The listing builds one solid part. Answer for the finished solid, in the listing's coordinates (mm). Face numbers are marked on the shaded views. A direction names the side the tool comes from. Give positions to 0.01 mm unless a question says otherwise; leave off trailing zeros. Order: outer loops, then holes, each group sorted by start corner. A loop starts at its lowest first (then second) coordinate and runs counter-clockwise, first axis right, second up. Notation, with made-up numbers: (46.5, -9) - (104.5, -9) arc R16 cw to (104.5, 0) - close; hole circle Ø10 at (40.25, 4). An arc over 180 degrees is marked (long way). Write each question's results on one line, items separated by ' | '. Start each with the question number.
1. Section D-D (x = 5) is taken. Give the vertices of the cut face in (y, z), and give its area (3 significant figures).
2. Determine the mould class of the marked faces 5, 6 and 7 for opening direction X: released by +X, released by -X, zero draft, split by the parting line, or undercut.
3. Find the intervals of material crossed by L1, parallel to Y at x = 0, z = 5.9; L2, parallel to X at y = 0, z = -9; L3, parallel to Z at x = -5.5, y = 4.5, in increasing order.
4. Section A-A (y = 0) is taken. Give the vertices of the cut face in (x, z), and give its area (3 significant figures).
5. Section C-C (z = -8) is taken. Give the vertices of the cut face in (x, y).
6. Section B-B (x = 0) is taken. Give the vertices of the cut face in (y, z).
7. Flat-ended cylindrical pins translate along their axes: pin 1 (4 mm diameter, centred on x = -4, z = -12.5, fed in from -Y); pin 2 (10 mm diameter, centred on x = -1.5, z = -9, fed in from +Y); pin 3 (4.5 mm diameter, centred on x = 0, y = 0, fed in from +Z). Find the tip coordinate at first contact, or state that the pin passes through.
8. Which of the six approach directions +Z, -Z, +X, -X, +Y, -Y give full straight-line access (tool end or side, diameter ignored) to the marked faces 1, 2, 3 and 4?
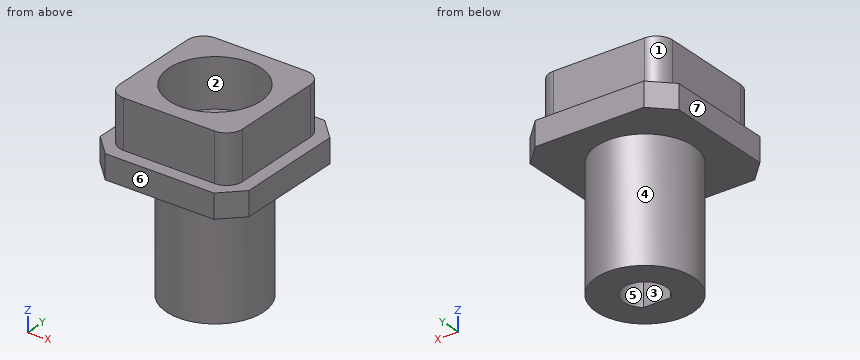
from build123d import *

# Parameters (mm, degrees)
PAD_DEPTH    = 3
SKETCH001_W  = 15.3
SKETCH001_H  = 15.3
SKETCH001_R  = 5.7
PAD001_DEPTH = 6
SKETCH002_R  = 6
PAD002_DEPTH = 15
POCKET_DEPTH = 24.001
FILLET_R     = 2


with BuildPart() as part:
    # Sketch → Pad (new body)
    with BuildSketch(Plane.XY):
        Polygon((-9.25, 6.75), (-6.75, 9.25), (6.75, 9.25), (9.25, 6.75), (9.25, -6.75), (6.75, -9.25), (-6.75, -9.25), (-9.25, -6.75), align=None)
    extrude(amount=PAD_DEPTH)

    # Sketch001 → Pad001 (new body)
    with BuildSketch(Plane.XY.offset(3)):
        Rectangle(SKETCH001_W, SKETCH001_H)
        Circle(SKETCH001_R, mode=Mode.SUBTRACT)
    extrude(amount=PAD001_DEPTH)

    # Sketch002 → Pad002 (new body)
    with BuildSketch(Plane(origin=(0, 0, 0), x_dir=(1, 0, 0), z_dir=(0, 0, -1))):
        Circle(SKETCH002_R)
    extrude(amount=PAD002_DEPTH)

    # Sketch003 → Pocket (cut, through all)
    with BuildSketch(Plane(origin=(0, 0, -15), x_dir=(1, 0, 0), z_dir=(0, 0, -1))):
        with BuildLine():
            Line((-1.684191, 2.02), (1.684191, 2.02))
            ThreePointArc((-1.684191, 2.02), (0, -2.63), (1.684191, 2.02))
        make_face()
    extrude(amount=-POCKET_DEPTH, mode=Mode.SUBTRACT)

    # Fillet
    fillet_edges = [part.edges().sort_by_distance(p)[0] for p in [
        (-7.65, -7.65, 6),
        (7.65, -7.65, 6),
        (-7.65, 7.65, 6),
        (7.65, 7.65, 6),
    ]]
    fillet(fillet_edges, radius=FILLET_R)


solid = part.part
Reported:
1) outline: (-9.25, 0) - (-3.32, 0) - (-3.32, -15) - (3.32, -15) - (3.32, 0) - (9.25, 0) - (9.25, 3) - (7.65, 3) - (7.65, 9) - (2.74, 9) - (2.74, 3) - (-2.74, 3) - (-2.74, 9) - (-7.65, 9) - (-7.65, 3) - (-9.25, 3) - close | area: 214 mm²
2) face 5: undercut | face 6: zero draft | face 7: released by -X
3) L1: -7.65 to -5.7, 5.7 to 7.65 | L2: -6 to -2.63, 2.63 to 6 | L3: 0 to 9
4) outline: (-9.25, 0) - (-6, 0) - (-6, -15) - (-2.63, -15) - (-2.63, 3) - (-5.7, 3) - (-5.7, 9) - (-7.65, 9) - (-7.65, 3) - (-9.25, 3) - close; (2.63, -15) - (6, -15) - (6, 0) - (9.25, 0) - (9.25, 3) - (7.65, 3) - (7.65, 9) - (5.7, 9) - (5.7, 3) - (2.63, 3) - close | area: 164 mm²
5) outline: circle Ø12 at (0, 0); hole (-1.68, -2.02) - (1.68, -2.02) arc R2.63 ccw (long way) to start
6) outline: (-9.25, 0) - (-6, 0) - (-6, -15) - (-2.02, -15) - (-2.02, 3) - (-5.7, 3) - (-5.7, 9) - (-7.65, 9) - (-7.65, 3) - (-9.25, 3) - close; (2.63, -15) - (6, -15) - (6, 0) - (9.25, 0) - (9.25, 3) - (7.65, 3) - (7.65, 9) - (5.7, 9) - (5.7, 3) - (2.63, 3) - close
7) pin 1: y = -5.66 | pin 2: y = 6 | pin 3: z = 3
8) face 1: +Z, -X, +Y | face 2: +Z | face 3: +Z, -Z | face 4: -Z
